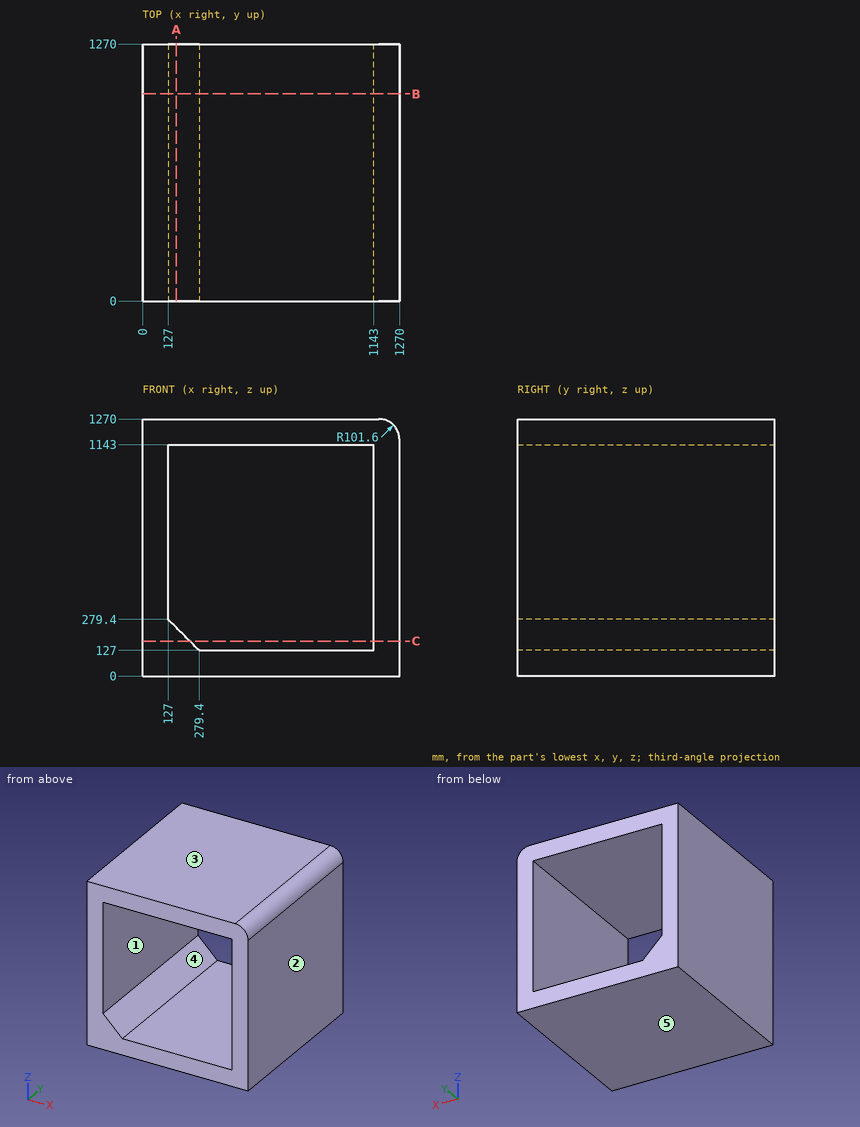
Check sheet for the drawn part. Datum: minimum x, y, z corner. Units: mm. A direction names the side the tool comes from. Round coordinates to 2 decimals unless told otherwise and drop trailing zeros. Order: outer loops, then holes, each group sorted by start corner. A loop starts at its lowest first (then second) coordinate and runs counter-clockwise, first axis right, second up. Notation, with made-up numbers: M 46.5,19.5 L 64.5,19.5 A21 cw 64.5,32.5 Z; hole C 71.5,38 d5. An arc over 180 degrees is marked long. Write each question's results on one line, items separated by ' | '. Start each with the question number.
1. Cross-section at A-A on x = 167. Record the boundary of the cut face in (y, z).
2. Material ranges on L1, parallel to X at y = 762, z = 435.5; L2, parallel to Z at x = 136, y = 585, recorded low to high. Write a range as from..to.
3. Cross-section at C-C on z = 172.5. Record the boundary of the cut face in (x, y).
4. Draft check along Z on the marked faces 1, 2 and 3. Enter one of: pulls with the +Z half, pulls with the -Z half, needs draft (parallel to the pull), parting line crosses it, or undercut.
5. Cross-section at B-B on y = 1023. Record the boundary of the cut face in (x, z), plus the area to 3 significant figures.
6. Set-up check for the marked faces 4 and 5: record each of +Z, -Z, +X, -X, +Y, -Y from which the full face is reachable in a straight line by a thin tool's end or side.
Resolved:
1) outline: M 0,0 L 1270,0 L 1270,239.4 L 0,239.4 Z; M 0,1143 L 1270,1143 L 1270,1270 L 0,1270 Z
2) L1: 0..127, 1143..1270 | L2: 0..270.4, 1143..1270
3) outline: M 0,0 L 233.9,0 L 233.9,1270 L 0,1270 Z; M 1143,0 L 1270,0 L 1270,1270 L 1143,1270 Z
4) face 1: undercut | face 2: needs draft | face 3: pulls with the +Z half
5) outline: M 0,0 L 1270,0 L 1270,1168.4 A101.6 ccw 1168.4,1270 L 0,1270 Z; hole M 127,279.4 L 279.4,127 L 1143,127 L 1143,1143 L 127,1143 Z | area: 590,000 mm2
6) face 4: +Y, -Y | face 5: -Z, +X, -X, +Y, -Y
